The model under review builds one solid part; all positions refer to its coordinate system, in mm. Round coordinates to 2 decimals unless told otherwise and drop trailing zeros. Write each loop counter-clockwise with the first axis right and the second up, starting at its lowest first coordinate (ties: lowest second). Pieces come first, ordered by that corner, then holes. Notation, with made-up numbers: (15, -35) -> (55, -35) arc R20 ccw to (55, -26) -> close; hole circle Ø4 at (8.25, 6). An arc over 180 degrees is marked (long way). Answer as a JSON object with one key per item and string values. Group by question number.
1) We need section B-B, the plane y = 13. Write out the cut boundary in (x, z), then the cut area to 3 significant figures.
2) Insertion check: pin 1 Ø8 at (x, z) = (20, 11.5) entering from +Y; pin 2 Ø6 at (x, y) = (15, 12) entering from -Z. Each pin has a flat end and moves straight along its axis. Give the tip position at first contact, or say it passes through.
3) To check wall thickness, follow probe 1 along Y at (x, z) = (31.5, -35); probe 2 along Z at (x, y) = (-18, 3); probe 3 along Z at (x, y) = (18, 24). State the ranges of each line that lie inside material, in increasing order. Write a range as [from, to].
4) We need section A-A, the plane x = 39. Write out the cut boundary in (y, z), then the cut area to 3 significant figures.
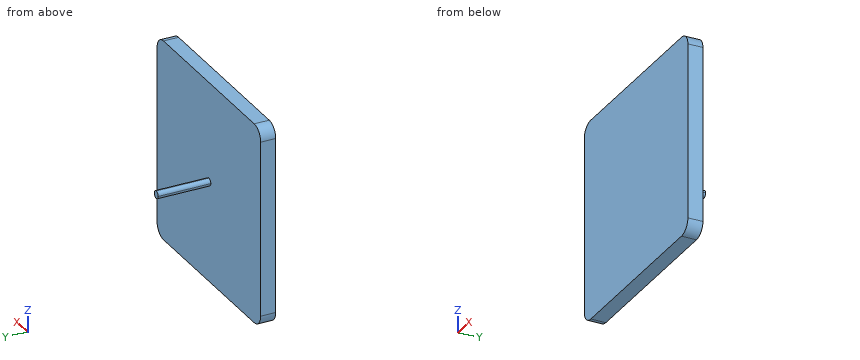
from build123d import *

# Parameters (mm, degrees)
SKETCH1_W                = 80
SKETCH1_H                = 80
BOSS_EXTRUDE1_DEPTH      = 6
FILLET1_R                = 5
BOSS_EXTRUDE2_DEPTH      = 21
BOSS_EXTRUDE2_DEPTH_BACK = 3


with BuildPart() as part:
    # Sketch1 → Boss-Extrude1 (new body)
    with BuildSketch(Plane(origin=(0, 0, 0), x_dir=(1, 0, 0), z_dir=(0, 1, 0))):
        with Locations((18.575784079, 13.984880667)):
            Rectangle(SKETCH1_W, SKETCH1_H)
    extrude(amount=BOSS_EXTRUDE1_DEPTH)

    # Fillet1
    fillet1_edges = [part.edges().sort_by_distance(p)[0] for p in [
        (-21.424215921, 3, -53.984880667),
        (58.575784079, 3, -53.984880667),
        (58.575784079, 3, 26.015119333),
        (-21.424215921, 3, 26.015119333),
    ]]
    fillet(fillet1_edges, radius=FILLET1_R)

    # Sketch3 → Boss-Extrude2 (add, two sides: drawn at the far end of the back side and taken through both)
    with BuildSketch(Plane(origin=(0, 6, 0), x_dir=(1, 0, 0), z_dir=(0, 1, 0)).offset(-BOSS_EXTRUDE2_DEPTH_BACK)):
        with BuildLine():
            ThreePointArc((20.075784079, 13.984880667), (19.63644425, 15.045540839), (18.575784079, 15.484880667))
            Line((18.575784079, 15.484880667), (18.575784079, 13.984880667))
            Line((18.575784079, 13.984880667), (20.075784079, 13.984880667))
        make_face()
        with BuildLine():
            Line((18.575784079, 13.984880667), (18.575784079, 15.484880667))
            ThreePointArc((18.575784079, 15.484880667), (17.515123907, 15.045540839), (17.075784079, 13.984880667))
            Line((17.075784079, 13.984880667), (18.575784079, 13.984880667))
        make_face()
        with BuildLine():
            Line((20.075784079, 13.984880667), (18.575784079, 13.984880667))
            Line((18.575784079, 13.984880667), (18.575784079, 12.484880667))
            ThreePointArc((18.575784079, 12.484880667), (19.63644425, 12.924220495), (20.075784079, 13.984880667))
        make_face()
        with BuildLine():
            Line((18.575784079, 12.484880667), (18.575784079, 13.984880667))
            Line((18.575784079, 13.984880667), (17.075784079, 13.984880667))
            ThreePointArc((17.075784079, 13.984880667), (17.515123907, 12.924220495), (18.575784079, 12.484880667))
        make_face()
    extrude(amount=BOSS_EXTRUDE2_DEPTH + BOSS_EXTRUDE2_DEPTH_BACK)


solid = part.part
Here are the results:
{
 "1": {"outline": "circle Ø3 at (18.58, -13.98)", "area": "7.07 mm^2"},
 "2": {"pin 1": "stops at y = 6", "pin 2": "stops at z = -15.37"},
 "3": {"probe 1": "y = [0, 6]", "probe 2": "z = [-53.73, 25.76]", "probe 3": "z = [-15.37, -12.6]"},
 "4": {"outline": "(0, -53.98) -> (6, -53.98) -> (6, 26.02) -> (0, 26.02) -> close", "area": "480 mm^2"}
}
